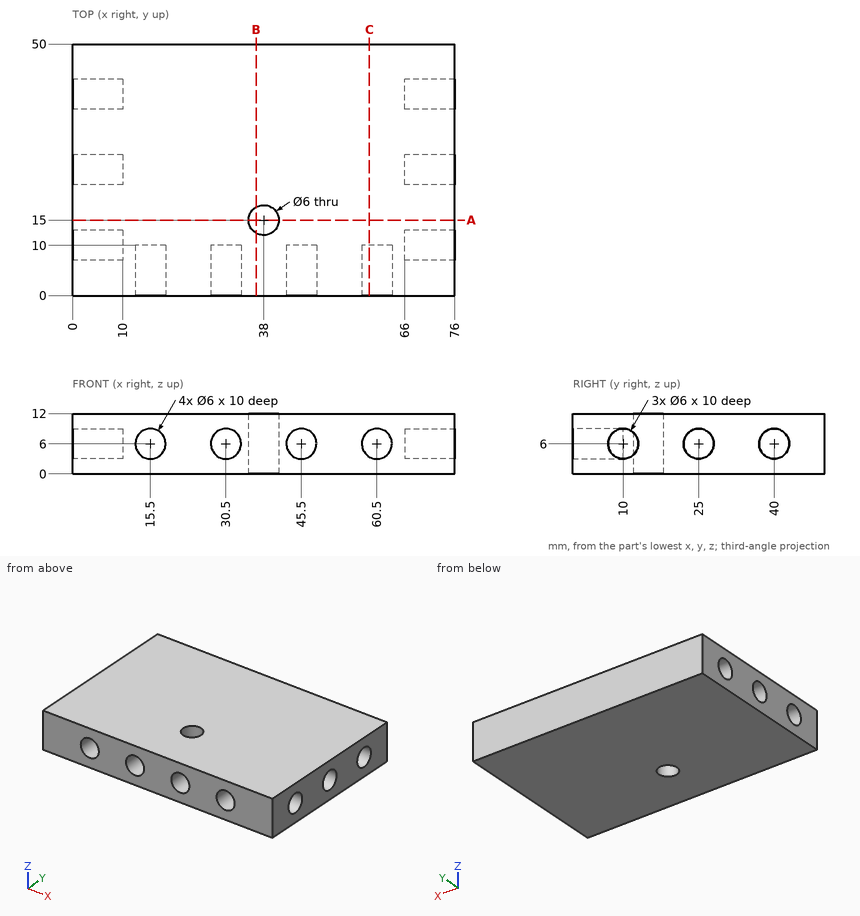
Verification items for this drawing (mm, ordinates from the low corner). Coordinates: 2 decimals unless noted, no trailing zeros. Order: outer loops, then holes, each group sorted by start corner. A loop starts at its lowest first (then second) coordinate and runs counter-clockwise, first axis right, second up.
Q1. Thickness scan on probe 1 along Y at (x, z) = (6.5, 6); probe 2 along Z at (x, y) = (69, 10); probe 3 along X at (y, z) = (7.5, 6). Record the ranges inside material, lowest first.
Reply:
probe 1: y = 0 to 7, 13 to 22, 28 to 37, 43 to 50
probe 2: z = 0 to 3, 9 to 12
probe 3: x = 10 to 12.5, 18.5 to 27.5, 33.5 to 42.5, 48.5 to 57.5, 63.5 to 66
Q2. Sectioned sample at B-B on x = 36.5. Record the cut outline in (y, z), and give its area (3 significant figures).
Reply:
outline: (0, 0) - (12.4, 0) - (12.4, 12) - (0, 12) - close; (17.6, 0) - (50, 0) - (50, 12) - (17.6, 12) - close
area: 538 mm2
Q3. Sectioned sample at A-A on y = 15. Record the cut outline in (x, z).
Reply:
outline: (0, 0) - (35, 0) - (35, 12) - (0, 12) - close; (41, 0) - (76, 0) - (76, 12) - (41, 12) - close
Q4. Depth check by flat-ended pin: pin 1 Ø3.5 at (y, z) = (40, 6) entering from +X; pin 2 Ø3 at (x, z) = (59.5, 6) entering from -Y; pin 3 Ø5.5 at (y, z) = (40, 6) entering from -X. Enter the tip coordinate at first touch or a pass-through.
Reply:
pin 1: stops at x = 66
pin 2: stops at y = 10
pin 3: stops at x = 10
Q5. Sectioned sample at C-C on x = 59. Record the cut outline in (y, z), and give its area (3 significant figures).
Reply:
outline: (0, 0) - (50, 0) - (50, 12) - (0, 12) - (0, 8.6) - (10, 8.6) - (10, 3.4) - (0, 3.4) - close
area: 548 mm2
